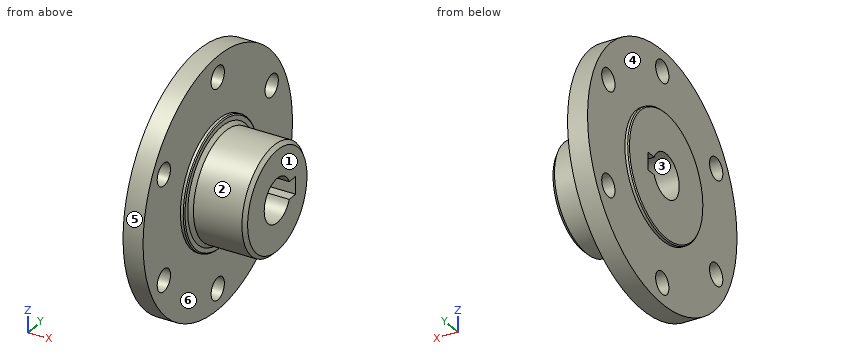
from build123d import *

# Parameters (mm, degrees)
SKETCH1_W                  = 4.572
SKETCH1_H                  = 28.575
SKETCH2_R                  = 14.2875
BOSS_EXTRUDE1_DEPTH        = 0.889
SKETCH3_R                  = 12.1666
BOSS_EXTRUDE2_DEPTH        = 12.7
SKETCH4_R                  = 14.2875
BOSS_EXTRUDE3_DEPTH        = 0.889
CUT_EXTRUDE1_DEPTH         = 20.05
SKETCH6_W                  = 19.05
SKETCH6_H                  = 5
F_10_CLEARANCE_HOLE1_D     = 5.08
F_10_CLEARANCE_HOLE1_DEPTH = 18.161
CHAMFER1_SIZE              = 0.254
CHAMFER2_SIZE              = 0.8128


with BuildPart() as part:
    # Sketch1 → Revolve1 (revolve)
    with BuildSketch(Plane(origin=(0, 0, 0), x_dir=(-1, 0, 0), z_dir=(0, 0, -1))):
        with Locations((15.321066246, 14.2875)):
            Rectangle(SKETCH1_W, SKETCH1_H)
    revolve(axis=Axis((-13.035066246, 0, 0), (-1, 0, 0)))

    # Sketch2 → Boss-Extrude1 (add)
    with BuildSketch(Plane(origin=(-13.035066246, 0, 0), x_dir=(0, 0, -1), z_dir=(1, 0, 0))):
        Circle(SKETCH2_R)
    extrude(amount=BOSS_EXTRUDE1_DEPTH)

    # Sketch3 → Boss-Extrude2 (add)
    with BuildSketch(Plane(origin=(-12.146066246, 0, 0), x_dir=(0, 0, -1), z_dir=(1, 0, 0))):
        Circle(SKETCH3_R)
    extrude(amount=BOSS_EXTRUDE2_DEPTH)

    # Sketch4 → Boss-Extrude3 (add)
    with BuildSketch(Plane.ZY.offset(17.607066246)):
        Circle(SKETCH4_R)
    extrude(amount=BOSS_EXTRUDE3_DEPTH)

    # Sketch5 → Cut-Extrude1 (cut, through all)
    with BuildSketch(Plane.ZY.offset(18.496066246)):
        with BuildLine():
            Line((2, 4.582575695), (2, 7))
            Line((2, 7), (-2, 7))
            Line((-2, 7), (-2, 4.582575695))
            ThreePointArc((-2, 4.582575695), (0, 5), (2, 4.582575695))
        make_face()
    extrude(amount=-CUT_EXTRUDE1_DEPTH, mode=Mode.SUBTRACT)

    # Sketch6 → Cut-Revolve1 (revolve, cut)
    with BuildSketch(Plane(origin=(0, 0, 0), x_dir=(-1, 0, 0), z_dir=(0, 0, -1))):
        with Locations((8.971066246, 2.5)):
            Rectangle(SKETCH6_W, SKETCH6_H)
    revolve(axis=Axis((0.553933754, 0, 0), (-1, 0, 0)), mode=Mode.SUBTRACT)

    # #10 Clearance Hole1
    with Locations(Plane.ZY.offset(17.607066246)):
        with Locations((11.90625, 20.622229928), (-11.90625, 20.622229928), (-23.8125, 0), (-11.90625, -20.622229928), (11.90625, -20.622229928), (23.8125, 0)):
            Hole(F_10_CLEARANCE_HOLE1_D / 2, depth=F_10_CLEARANCE_HOLE1_DEPTH)

    # Chamfer1
    chamfer1_edges = [part.edges().sort_by_distance(p)[0] for p in [
        (-18.496066246, 0, -14.2875),
        (-12.146066246, 0, 14.2875),
    ]]
    chamfer(chamfer1_edges, length=CHAMFER1_SIZE)

    # Chamfer2
    chamfer2_edges = [part.edges().sort_by_distance(p)[0] for p in [
        (-12.146066246, 0, 12.1666),
        (0.553933754, 0, 12.1666),
    ]]
    chamfer(chamfer2_edges, length=CHAMFER2_SIZE)


solid = part.part
Can you work these out from the model? Positions are in its coordinate system, mm. Face numbers are marked on the shaded views. A direction names the side the tool comes from. Coordinates: 2 decimals unless noted, no trailing zeros. Loops run counter-clockwise (first coordinate to the right, second up) from the corner with the lowest first, then second, coordinate; pieces in that order, holes last. Notation, with made-up numbers: M 55,-38 L 89,-38 A33 cw 89,0 Z; hole C 51.25,52.5 d3. An arc over 180 degrees is marked long. Return JSON: item names as keys, results as strings. Group by question number.
Item 1: Thinking about a two-plate mould opening in Y: for the marked faces 1, 2 and 3, which applies, released by +Y, released by -Y, zero draft, split by the parting line, or undercut?
Item 2: Imagine slicing it at B-B (x = -8.75). Please give me the cut outline in (y, z), and give its area (3 significant figures).
Item 3: If I drill on L1, parallel to Z at x = -14.75, y = 21; L2, parallel to Y at x = -17.25, z = 13; L3, parallel to X at y = -24, z = 7, over which ranges is the centre line in solid material (lowest first)? Write a range as from..to.
Item 4: Imagine slicing it at C-C (y = 0). Give the number of separate pieces and of enclosed holes in the cut face, and give its area (3 significant figures).
Item 5: On a 3-axis mill with a long thin cutter (end or side, diameter ignored), from which of +Z, -Z, +X, -X, +Y, -Y can I reach the whole of each face in a straight line? I mean the marked faces 4, 5 and 6. Say none if no direction works.
Item 6: I'm going to push flat-ended pins straight in: pin 1 Ø5 at (y, z) = (19.5, 12) entering from -X; pin 2 Ø8 at (x, y) = (-8, -6.5) entering from -Z; pin 3 Ø2.5 at (x, y) = (-10, 6) entering from +Z. Where does each tip first touch, or does it pass through?
Verdict:
{
 "1": {"face 1": "zero draft", "face 2": "split by the parting line", "face 3": "undercut"},
 "2": {"outline": "C 0,0 d24.33; hole M 4.58,-2 L 7,-2 L 7,2 L 4.58,2 A5 ccw long Z", "area": "378 mm^2"},
 "3": {"L1": "z = -19.38..-14.42, -9.39..9.39, 14.42..19.38", "L2": "y = -25.45..-22.91, -18.33..18.33, 22.91..25.45", "L3": "x = -17.61..-13.04"},
 "4": {"separate pieces": "4", "enclosed holes": "0", "area": "384 mm^2"},
 "5": {"face 4": "-X", "face 5": "+X, -X", "face 6": "+X"},
 "6": {"pin 1": "stops at x = -17.61", "pin 2": "stops at z = -11.91", "pin 3": "stops at z = 11.2"}
}
